```python
from build123d import *

# Parameters (mm, degrees)
SKETCH_1_W          = 74
SKETCH_1_H          = 74
EXTRUDE_1_DEPTH     = 2
SKETCH_2_R          = 15
CUT_EXTRUDE_1_DEPTH = 2
M3X0_5_1_D          = 2.5


with BuildPart() as part:
    # ｽｹｯﾁ1 → ﾎﾞｽ - 押し出し1 (new body)
    with BuildSketch(Plane.XY):
        with Locations((37, 37)):
            Rectangle(SKETCH_1_W, SKETCH_1_H)
    extrude(amount=EXTRUDE_1_DEPTH)

    # ｽｹｯﾁ2 → ｶｯﾄ - 押し出し1 (cut)
    with BuildSketch(Plane.XY.offset(2)):
        with Locations((37, 37)):
            Circle(SKETCH_2_R)
    extrude(amount=-CUT_EXTRUDE_1_DEPTH, mode=Mode.SUBTRACT)

    # M3x0.5 ねじ穴1 (through all)
    with Locations(Plane.XY.offset(2)):
        with Locations((7, 67), (67, 67)):
            m3x0_5_1 = Hole(M3X0_5_1_D / 2)

    # ﾐﾗｰ1: M3x0.5 ねじ穴1 across plane
    add(m3x0_5_1.mirror(Plane.ZX.offset(37)), mode=Mode.SUBTRACT)


solid = part.part
```
Geometry: final body of the model. Coordinates: model frame, mm. Round coordinates to 2 decimals unless told otherwise and drop trailing zeros. Write each loop counter-clockwise with the first axis right and the second up, starting at its lowest first coordinate (ties: lowest second). Pieces come first, ordered by that corner, then holes.
Item 1: Section query A-A (x = 67). Return loops of the section in (y, z), plus the area to 3 significant figures.
Item 2: Mould query, pull axis Y, two halves, no side actions, for faces 1 (the face through (36, 74, 1)), 2 (the face through (66.328, 68.054, 0.986)), 3 (the face through (36, 21, 2)). Classes: +Y half, -Y half, draft (parallel to the pull), parting line (faces both ways), or undercut.
Item 3: Section query C-C (y = 37). Return loops of the section in (x, z), plus the area to 3 significant figures.
Item 4: Section query B-B (z = 1.7). Return loops of the section in (x, y).
Item 5: Section query D-D (x = 25). Return loops of the section in (y, z), plus the area to 3 significant figures.
Item 6: Material intervals for L1, parallel to Y at x = 67, z = 0.9; L2, parallel to Y at x = 37, z = 1.1, sorted ascending.
Completed:
1. outline: (0, 0) - (5.75, 0) - (5.75, 2) - (0, 2) - close; (8.25, 0) - (65.75, 0) - (65.75, 2) - (8.25, 2) - close; (68.25, 0) - (74, 0) - (74, 2) - (68.25, 2) - close
1. area: 138 mm2
2. face 1: +Y half
2. face 2: undercut
2. face 3: draft
3. outline: (0, 0) - (22, 0) - (22, 2) - (0, 2) - close; (52, 0) - (74, 0) - (74, 2) - (52, 2) - close
3. area: 88.0 mm2
4. outline: (0, 0) - (74, 0) - (74, 74) - (0, 74) - close; hole circle Ø2.5 at (7, 7); hole circle Ø2.5 at (7, 67); hole circle Ø30 at (37, 37); hole circle Ø2.5 at (67, 7); hole circle Ø2.5 at (67, 67)
5. outline: (0, 0) - (28, 0) - (28, 2) - (0, 2) - close; (46, 0) - (74, 0) - (74, 2) - (46, 2) - close
5. area: 112 mm2
6. L1: y = 0 to 5.75, 8.25 to 65.75, 68.25 to 74
6. L2: y = 0 to 22, 52 to 74
